from build123d import *

# Parameters (mm, degrees)
SKETCH1_R           = 3.8
BOSS_EXTRUDE1_DEPTH = 2.2
SKETCH2_R           = 2
BOSS_EXTRUDE2_DEPTH = 8
CHAMFER1_SIZE       = 0.3
CUT_EXTRUDE1_DEPTH  = 2
FILLET1_R           = 1.8


with BuildPart() as part:
    # Sketch1 → Boss-Extrude1 (new body)
    with BuildSketch(Plane.XY):
        Circle(SKETCH1_R)
    extrude(amount=BOSS_EXTRUDE1_DEPTH)

    # Sketch2 → Boss-Extrude2 (add)
    with BuildSketch(Plane(origin=(0, 0, 0), x_dir=(-1, 0, 0), z_dir=(0, 0, -1))):
        Circle(SKETCH2_R)
    extrude(amount=BOSS_EXTRUDE2_DEPTH)

    # Chamfer1
    chamfer1_edges = [part.edges().sort_by_distance(p)[0] for p in [
        (2, 0, -8),
    ]]
    chamfer(chamfer1_edges, length=CHAMFER1_SIZE)

    # Sketch3 → Cut-Extrude1 (cut)
    with BuildSketch(Plane.XY.offset(2.2)):
        Polygon((0, 1.443375673), (-1.25, 0.721687836), (-1.25, -0.721687836), (0, -1.443375673), (1.25, -0.721687836), (1.25, 0.721687836), align=None)
    extrude(amount=-CUT_EXTRUDE1_DEPTH, mode=Mode.SUBTRACT)

    # Fillet1
    fillet1_edges = [part.edges().sort_by_distance(p)[0] for p in [
        (-3.8, 0, 2.2),
    ]]
    fillet(fillet1_edges, radius=FILLET1_R)


solid = part.part
Could you check a few things on this model? Use its own coordinates, in mm. A direction names the side the tool comes from. Coordinates: 2 decimals unless noted, no trailing zeros. Order: outer loops, then holes, each group sorted by start corner. A loop starts at its lowest first (then second) coordinate and runs counter-clockwise, first axis right, second up.
Q1. Will these pins go through, and if not, where does the flat tip stop? pin 1 (1.5 mm diameter, centred on x = 0, y = -0.5, fed in from +Z); pin 2 (3 mm diameter, centred on x = 3, z = -6.5, fed in from -Y); pin 3 (4 mm diameter, centred on y = -2.5, z = -3.5, fed in from -X).
Q2. Thinking about a two-plate mould opening in Y: for faces 4 (the cylindrical face through (0, -2, -4)), 5 (the flat face through (1.25, 0, 1)), 6 (the flat face through (0, 0, -8)), which applies, released by +Y, released by -Y, zero draft, split by the parting line, or undercut?
Q3. Suppose I cut it at A-A on y = 0. Please give me the cut outline in (x, z), and give its area (3 significant figures).
Q4. Which directions (+Z, -Z, +X, -X, +Y, -Y) give clear straight access to the entire face, cutting with the end or side of a thin tool? Please do faces 1 (the flat face through (2, -2, 0)), 2 (the flat face through (-0.616, 1.088, 1.214)), 3 (the cylindrical face through (-3.796, 0.167, 0.197)).
Q5. Suppose I cut it at B-B on z = -6. Please give me the cut outline in (x, y).
Q6. Please list where these lines run through material, in increasing order: L1, parallel to Y at x = -1, z = 1; L2, parallel to Z at x = 0, y = 0.5; L3, parallel to Y at x = 0.5, z = -4.25.
Answer:
1. pin 1: stops at z = 0.2
1. pin 2: stops at y = -1.32
1. pin 3: stops at x = -1.94
2. face 4: split by the parting line
2. face 5: undercut
2. face 6: zero draft
3. outline: (-3.8, 0) - (-2, 0) - (-2, -7.7) - (-1.7, -8) - (1.7, -8) - (2, -7.7) - (2, 0) - (3.8, 0) - (3.8, 0.4) arc R1.8 ccw to (2, 2.2) - (1.25, 2.2) - (1.25, 0.2) - (-1.25, 0.2) - (-1.25, 2.2) - (-2, 2.2) arc R1.8 ccw to (-3.8, 0.4) - close
3. area: 42.2 mm2
4. face 1: -Z
4. face 2: +Z
4. face 3: +Z, -Z
5. outline: circle Ø4 at (0, 0)
6. L1: y = -3.56 to -0.87, 0.87 to 3.56
6. L2: z = -8 to 0.2
6. L3: y = -1.94 to 1.94
